The listing builds one solid part. Answer for the finished solid, in the listing's coordinates (mm). Face numbers are marked on the shaded views. A direction names the side the tool comes from. Coordinates: 2 decimals unless noted, no trailing zeros. Write each loop counter-clockwise with the first axis right and the second up, starting at its lowest first coordinate (ties: lowest second). Pieces come first, ordered by that corner, then holes. Notation, with made-up numbers: M 23,81 L 75,81 A12 cw 75,101 Z; hole C 73.25,41 d4. An arc over 180 degrees is marked long. Answer as a JSON object with one key per item and string values. Group by question number.
from build123d import *

# Parameters (mm, degrees)
EXTRUDE015_DEPTH = 1
EXTRUDE014_DEPTH = 2.25


with BuildPart() as extrude015:
    # Sketch015 → Extrude015 (new body)
    with BuildSketch(Plane.XZ):
        with BuildLine():
            ThreePointArc((11.7, 16.35), (11.063604, 16.086396), (10.8, 15.45))
            Line((10.8, 14.2), (10.8, 15.45))
            ThreePointArc((10.8, 14.2), (11.23934, 13.13934), (12.3, 12.7))
            Line((16.8, 12.7), (12.3, 12.7))
            ThreePointArc((16.8, 12.7), (17.86066, 13.13934), (18.3, 14.2))
            Line((18.3, 15.45), (18.3, 14.2))
            ThreePointArc((18.3, 15.45), (18.036396, 16.086396), (17.4, 16.35))
            Line((11.7, 16.35), (17.4, 16.35))
        make_face()
    extrude(amount=EXTRUDE015_DEPTH)


with BuildPart() as extrude015_1:
    # Extrude015 placement: moved
    add(extrude015.part.moved(Location((0, 3, 0))))


with BuildPart() as button1:
    # Sketch014 → Extrude014 (new body)
    with BuildSketch(Plane.XZ):
        with BuildLine():
            ThreePointArc((12.3, 16.35), (11.663604, 16.086396), (11.4, 15.45))
            Line((11.4, 14.2), (11.4, 15.45))
            ThreePointArc((11.4, 14.2), (11.663604, 13.563604), (12.3, 13.3))
            Line((16.8, 13.3), (12.3, 13.3))
            ThreePointArc((16.8, 13.3), (17.436396, 13.563604), (17.7, 14.2))
            Line((17.7, 15.45), (17.7, 14.2))
            ThreePointArc((17.7, 15.45), (17.436396, 16.086396), (16.8, 16.35))
            Line((12.3, 16.35), (16.8, 16.35))
        make_face()
    extrude(amount=EXTRUDE014_DEPTH)


with BuildPart() as button1_1:
    # Extrude014 placement: moved
    add(button1.part.moved(Location((0, 2, 0))))

    # Fusion018: union Extrude015
    add(extrude015_1.part)


solid = button1_1.part
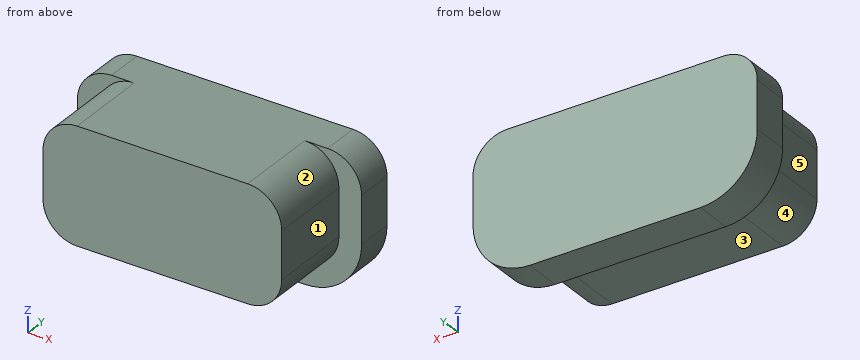
Item 1: A cutting plane is placed at C-C, the plane x = 14. Write down the section's boundary in (y, z), and give its area (3 significant figures).
Item 2: A tool of negligible diameter and unlimited length cuts with its end or side. For the marked faces 1, 2, 3, 4 and 5, from which of +Z, -Z, +X, -X, +Y, -Y can it reach the whole face along a straight path? Write none if from no direction.
Item 3: Consider L1, parallel to Z at x = 13.25, y = 0.8; L2, parallel to X at y = 0.95, z = 14.9; L3, parallel to X at y = 2.4, z = 13.7. Determine where each line is inside the solid, lowest interval first. Write a range as from..to.
Item 4: A cutting plane is placed at B-B, the plane z = 14.5. Write down the section's boundary in (x, y), and give its area (3 significant figures).
Item 5: Flat-ended cylindrical pins translate along their axes: pin 1 Ø1 at (y, z) = (0.5, 14.5) entering from +X; pin 2 Ø1 at (y, z) = (1, 15) entering from -X. Find the tip coordinate at first contact, or state that the pin passes through.
Item 6: A cutting plane is placed at A-A, the plane y = 2.3. Write down the section's boundary in (x, z), and give its area (3 significant figures).
Answer:
{
 "1": {"outline": "M -0.25,13.3 L 2,13.3 L 2,12.7 L 3,12.7 L 3,16.35 L -0.25,16.35 Z", "area": "10.5 mm2"},
 "2": {"face 1": "+Z, -Z, +X, -Y", "face 2": "+Z, +X, -Y", "face 3": "-Z, +X, -X, -Y", "face 4": "-Z, -X, -Y", "face 5": "+Z, -Z, -X, -Y"},
 "3": {"L1": "13.3..16.35", "L2": "11.4..17.7", "L3": "10.89..18.21"},
 "4": {"outline": "M 10.8,2 L 11.4,2 L 11.4,-0.25 L 17.7,-0.25 L 17.7,2 L 18.3,2 L 18.3,3 L 10.8,3 Z", "area": "21.7 mm2"},
 "5": {"pin 1": "x = 17.7", "pin 2": "x = 11.4"},
 "6": {"outline": "M 10.8,14.2 A1.5 ccw 12.3,12.7 L 16.8,12.7 A1.5 ccw 18.3,14.2 L 18.3,15.45 A0.9 ccw 17.4,16.35 L 11.7,16.35 A0.9 ccw 10.8,15.45 Z", "area": "26.1 mm2"}
}
